```python
from build123d import *

# Parameters (mm, degrees)
SKETCH1_R           = 2.45
SKETCH1_W           = 13.8
SKETCH1_H           = 239
BOSS_EXTRUDE1_DEPTH = 1
FILLET2_R           = 10


with BuildPart() as part:
    # Sketch1 → Boss-Extrude1 (new body)
    with BuildSketch(Plane(origin=(0, 0, 0), x_dir=(1, 0, 0), z_dir=(0, 1, 0))):
        Polygon((-39.9, -163.5), (-21.9, -163.5), (-21.9, -167.5), (-16.9, -167.5), (-16.9, -183.5), (16.9, -183.5), (16.9, -167.5), (21.9, -167.5), (21.9, -163.5), (39.9, -163.5), (39.9, 163.5), (21.9, 163.5), (21.9, 167.5), (16.9, 167.5), (16.9, 183.5), (-16.9, 183.5), (-16.9, 167.5), (-21.9, 167.5), (-21.9, 163.5), (-39.9, 163.5), align=None)
        with Locations(Location((-32.4, 127.5, 0), (0, 0, 270))):
            Circle(SKETCH1_R, mode=Mode.SUBTRACT)
        with Locations(Location((32.4, 127.5, 0), (0, 0, 270))):
            Circle(SKETCH1_R, mode=Mode.SUBTRACT)
        with Locations(Location((-32.4, -127.5, 0), (0, 0, 270))):
            Circle(SKETCH1_R, mode=Mode.SUBTRACT)
        with Locations(Location((32.4, -127.5, 0), (0, 0, 270))):
            Circle(SKETCH1_R, mode=Mode.SUBTRACT)
        with Locations(Location((-32.4, -157.5, 0), (0, 0, 270))):
            Circle(SKETCH1_R, mode=Mode.SUBTRACT)
        with Locations(Location((32.4, -157.5, 0), (0, 0, 270))):
            Circle(SKETCH1_R, mode=Mode.SUBTRACT)
        with Locations(Location((32.4, 157.5, 0), (0, 0, 270))):
            Circle(SKETCH1_R, mode=Mode.SUBTRACT)
        with Locations(Location((-32.4, 157.5, 0), (0, 0, 270))):
            Circle(SKETCH1_R, mode=Mode.SUBTRACT)
        with Locations(Location((0, 178.5, 0), (0, 0, 270))):
            Circle(SKETCH1_R, mode=Mode.SUBTRACT)
        with Locations(Location((0, -178.5, 0), (0, 0, 270))):
            Circle(SKETCH1_R, mode=Mode.SUBTRACT)
        Rectangle(SKETCH1_W, SKETCH1_H, mode=Mode.SUBTRACT)
    extrude(amount=BOSS_EXTRUDE1_DEPTH)

    # Fillet2
    # the kernel refuses this fillet: 10 mm, written as the material it adds along each edge
    with BuildSketch(Plane(origin=(6.9, 0, -119.5), x_dir=(-1, 0, 0), z_dir=(0, 1, 0)), Plane(origin=(6.9, 0, 119.5), x_dir=(0, 0, -1), z_dir=(0, 1, 0)), Plane(origin=(-6.9, 0, 119.5), x_dir=(1, 0, 0), z_dir=(0, 1, 0))) as fillet2_piece_1:
        with BuildLine():
            CenterArc((FILLET2_R, FILLET2_R), FILLET2_R, 180, 90)
            Line((0, FILLET2_R), (0, 0))
            Line((0, 0), (FILLET2_R, 0))
        make_face()
    extrude(amount=1)
    with BuildSketch(Plane(origin=(-6.9, 0, -119.5), x_dir=(1, 0, 0), z_dir=(0, 1, 0))) as fillet2_piece_2:
        with BuildLine():
            CenterArc((FILLET2_R, -FILLET2_R), FILLET2_R, 90, 90)
            Line((0, -FILLET2_R), (0, 0))
            Line((0, 0), (FILLET2_R, 0))
        make_face()
    extrude(amount=1)


solid = part.part
```
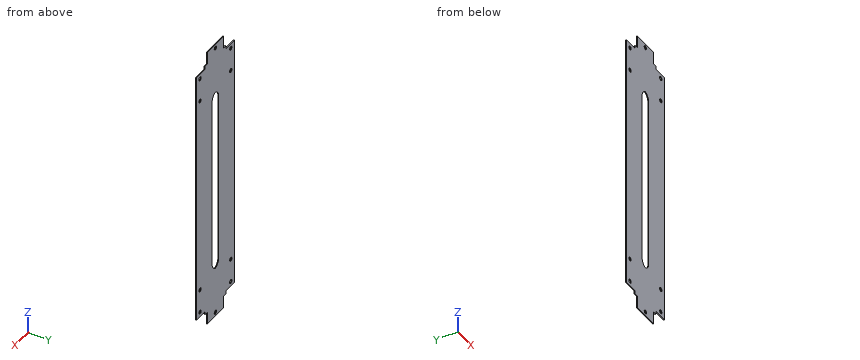
Source: CAD feature listing. Evaluate the final solid. Frame: model axes, mm. Round coordinates to 2 decimals unless told otherwise and drop trailing zeros. Loops run counter-clockwise (first coordinate to the right, second up) from the corner with the lowest first, then second, coordinate; pieces in that order, holes last. Notation, with made-up numbers: (54, 35) - (81, 35) arc R19 ccw to (81, 44) - close; hole circle Ø3 at (-3, 62.5). An arc over 180 degrees is marked (long way). Use CSV: the item, a comma, the result in double quotes.
Q1. Section query A-A, the plane z = 78.5. Output: boundary loops of the cut face in (x, y).
Reported:
outline,"(-39.9, 0) - (-6.9, 0) - (-6.9, 1) - (-39.9, 1) - close; (6.9, 0) - (39.9, 0) - (39.9, 1) - (6.9, 1) - close"
Q2. Ray query, line 1 along X through (y, z) = (0.5, 157.5); line 2 along Z through (x, y) = (-32, 0.5); line 3 along X through (y, z) = (0.15, 86.5). Return the intervals inside material, ascending.
Reported:
line 1,"-39.9 to -34.85, -29.95 to 29.95, 34.85 to 39.9"
line 2,"-163.5 to -159.92, -155.08 to -129.92, -125.08 to 125.08, 129.92 to 155.08, 159.92 to 163.5"
line 3,"-39.9 to -6.9, 6.9 to 39.9"
Q3. Pin query (flat end, axial travel): pin 1 Ø0.5 at (y, z) = (0.5, 165) entering from -X; pin 2 Ø6.5 at (x, z) = (-32.4, 127.5) entering from -Y; pin 3 Ø0.5 at (x, y) = (20, 0.5) entering from +Z; pin 4 Ø0.5 at (y, z) = (0.5, -178.5) entering from -X. Return the tip coordinate at first contact, or that it passes through.
Reported:
pin 1,"x = -21.9"
pin 2,"y = 0"
pin 3,"z = 167.5"
pin 4,"x = -16.9"
Q4. Section query B-B, the plane y = 0.2. Give the number of separate pieces and of enclosed holes in the cut face, then the cut area to 3 significant figures.
Reported:
separate pieces,"1"
enclosed holes,"11"
area,"24,100 mm^2"
